For this review, take the finished solid that the model builds, in its own axes (mm). A direction names the side the tool comes from. Give positions to 0.01 mm unless a question says otherwise; leave off trailing zeros. Write each loop counter-clockwise with the first axis right and the second up, starting at its lowest first coordinate (ties: lowest second). Pieces come first, ordered by that corner, then holes. Notation, with made-up numbers: (73, 63) -> (100, 63) arc R27 cw to (100, 96) -> close; hole circle Ø8 at (28, 58.5). An arc over 180 degrees is marked (long way). Answer as CSV lines item,"result".
```python
from build123d import *

# Parameters (mm, degrees)
SKETCH1_R               = 30
SKETCH1_R_2             = 2.1
BOSS_EXTRUDE1_DEPTH     = 5
SKETCH2_R               = 10.05
BOSS_EXTRUDE2_DEPTH     = 27
CUT_EXTRUDE1_DEPTH      = 20
CUT_EXTRUDE1_DEPTH_BACK = 20
SKETCH3_R               = 1.85


with BuildPart() as part:
    # Sketch1 → Boss-Extrude1 (new body)
    with BuildSketch(Plane.XY):
        Circle(SKETCH1_R)
        with Locations((0, 6.5)):
            Circle(SKETCH1_R_2, mode=Mode.SUBTRACT)
        with Locations((6, 0)):
            Circle(SKETCH1_R_2, mode=Mode.SUBTRACT)
        with Locations((0, -6.5)):
            Circle(SKETCH1_R_2, mode=Mode.SUBTRACT)
        with Locations((-6, 0)):
            Circle(SKETCH1_R_2, mode=Mode.SUBTRACT)
    extrude(amount=BOSS_EXTRUDE1_DEPTH)

    # Sketch2 → Boss-Extrude2 (add)
    with BuildSketch(Plane.XY.offset(5)):
        Circle(SKETCH2_R)
        with BuildLine():
            Line((-3.016620626, 4.05), (3.016620626, 4.05))
            ThreePointArc((3.016620626, 4.05), (0, -5.05), (-3.016620626, 4.05))
        make_face(mode=Mode.SUBTRACT)
        with BuildLine():
            ThreePointArc((1.327118589, 4.8725), (0, 4.4), (-1.327118589, 4.8725))
            ThreePointArc((-1.327118589, 4.8725), (0, 5.05), (1.327118589, 4.8725))
        make_face(mode=Mode.SUBTRACT)
    extrude(amount=BOSS_EXTRUDE2_DEPTH)

    # Sketch3 → Cut-Extrude1 (cut, two sides: drawn at the far end of the back side and taken through both)
    with BuildSketch(Plane(origin=(0, 4.05, 0), x_dir=(-1, 0, 0), z_dir=(0, -1, 0)).offset(-CUT_EXTRUDE1_DEPTH_BACK)):
        with Locations(Location((0, -22, 0), (0, 0, 270))):
            Circle(SKETCH3_R)
    extrude(amount=CUT_EXTRUDE1_DEPTH + CUT_EXTRUDE1_DEPTH_BACK, mode=Mode.SUBTRACT)


solid = part.part
```
Q1. Add section D-D (z = 22). Write out the cut boundary in (x, y).
Answer block:
outline,"(-3.02, 4.05) -> (-1.85, 4.05) -> (-1.85, 9.88) arc R10.05 ccw to (-1.85, -9.88) -> (-1.85, -4.7) arc R5.05 cw to start; (1.85, -9.88) arc R10.05 ccw to (1.85, 9.88) -> (1.85, 4.05) -> (3.02, 4.05) arc R5.05 cw to (1.85, -4.7) -> close"
Q2. Clearance check with flat-ended pins moving along their axes: pin 1 (1 mm diameter, centred on x = 6, y = -0.5, fed in from -Z); pin 2 (5 mm diameter, centred on x = 0, z = 22, fed in from +Y); pin 3 (5 mm diameter, centred on x = -19, y = 18, fed in from +Z). State where each tip first meets the part, or that it passes through.
Answer block:
pin 1,"stops at z = 5"
pin 2,"stops at y = 10.05"
pin 3,"stops at z = 5"
Q3. To check wall thickness, follow probe 1 along Z at (x, y) = (-4, -16); probe 2 along Y at (x, z) = (-3.5, 8.5); probe 3 along Y at (x, z) = (6, 1). State the ranges of each line that lie inside material, in increasing order. Write a range as [from, to].
Answer block:
probe 1,"z = [0, 5]"
probe 2,"y = [-9.42, -3.64], [3.64, 9.42]"
probe 3,"y = [-29.39, -2.1], [2.1, 29.39]"
Q4. For faces 1 (the cylindrical face through (0.71, 7.09, 23.71)), 2 (the flat face through (0, 0, 5)), 3 (the cylindrical face through (-8.1, 0.09, 2.46)), list the 3-axis set-ups (+Z, -Z, +X, -X, +Y, -Y) from which the entire face can be reached by the end or side of a thin tool; tool diameter is ignored.
Answer block:
face 1,"+Y, -Y"
face 2,"+Z"
face 3,"-Z"
Q5. Add section B-B (y = 0). Write out the cut boundary in (x, z).
Answer block:
outline,"(-30, 0) -> (-8.1, 0) -> (-8.1, 5) -> (-5.05, 5) -> (-5.05, 32) -> (-10.05, 32) -> (-10.05, 5) -> (-30, 5) -> close; (-3.9, 0) -> (3.9, 0) -> (3.9, 5) -> (-3.9, 5) -> close; (5.05, 5) -> (8.1, 5) -> (8.1, 0) -> (30, 0) -> (30, 5) -> (10.05, 5) -> (10.05, 32) -> (5.05, 32) -> close"
Q6. Draft analysis for pull direction X (two halves, no side actions). For faces 4 (the cylindrical face through (-29.97, 1.32, 2.46)), 5 (the flat face through (0, 4.05, 18)), 6 (the flat face through (0, 0, 0)), state which applies: released by +X, released by -X, zero draft, split by the parting line, or undercut.
Answer block:
face 4,"split by the parting line"
face 5,"undercut"
face 6,"zero draft"
Q7. Add section C-C (z = 26). Write out the cut boundary in (x, y).
Answer block:
outline,"circle Ø20.1 at (0, 0); hole (-3.02, 4.05) arc R5.05 ccw (long way) to (3.02, 4.05) -> close; hole (-1.33, 4.87) arc R2.1 ccw to (1.33, 4.87) arc R5.05 ccw to start"
Q8. Add section A-A (x = 0). State how many separate pieces and enclosed holes the cut face has, plus the area to 3 significant figures.
Answer block:
separate pieces,"6"
enclosed holes,"0"
area,"499 mm2"
